Here's the drawing with two shaded views (mm, measured from the low corner). I have some questions. A direction names the side the tool comes from. Round coordinates to 2 decimals unless told otherwise and drop trailing zeros. Loops run counter-clockwise (first coordinate to the right, second up) from the corner with the lowest first, then second, coordinate; pieces in that order, holes last. Notation, with made-up numbers: M 86,67 L 112,67 A24 ccw 112,92 Z; hole C -3,15.5 d1. An arc over 180 degrees is marked long. Answer as a JSON object with one key per item and string values.
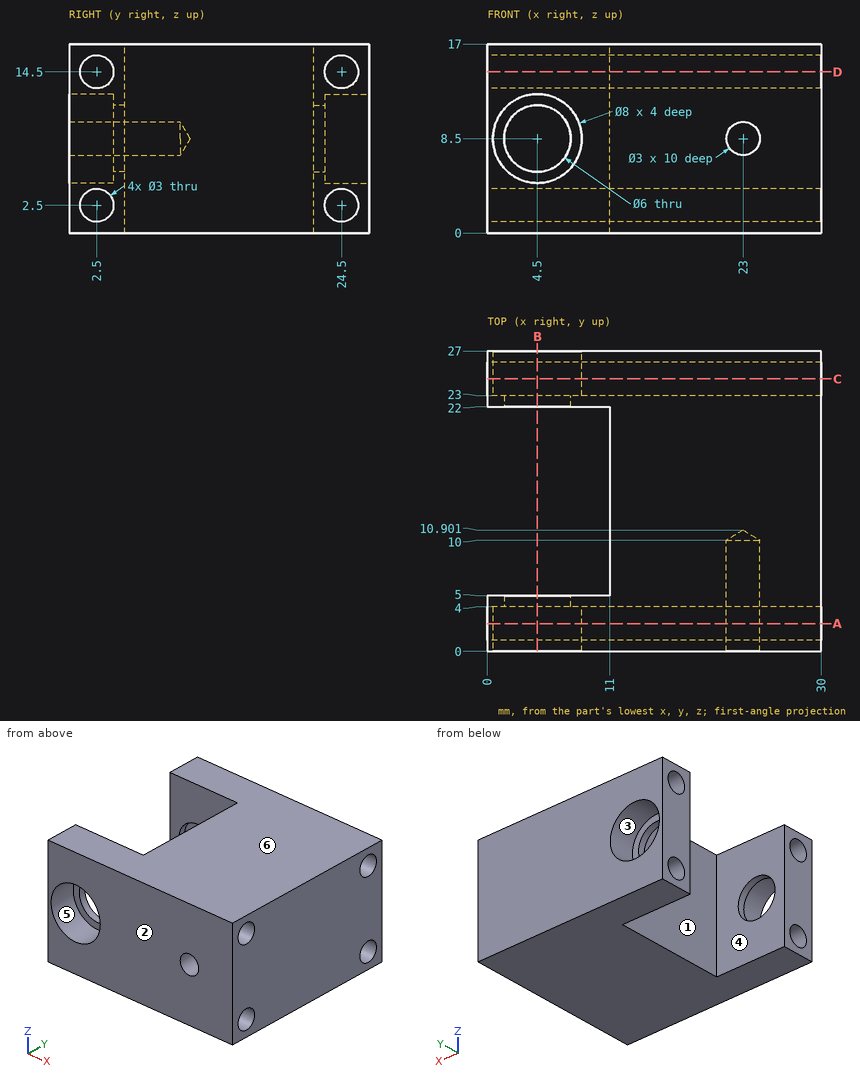
Item 1: We'd pull the mould along X, two halves only. Please class the marked faces 1, 2 and 3: +X half, -X half, draft (parallel to the pull), parting line (faces both ways), or undercut.
Solution:
{"face 1": "-X half", "face 2": "draft", "face 3": "undercut"}
Item 2: I want a section at B-B on x = 4.5. List the corners of the cut face in (y, z) for me.
Solution:
{"outline": "M 0,0 L 5,0 L 5,5.5 L 4,5.5 L 4,4.5 L 0,4.5 Z; M 0,12.5 L 4,12.5 L 4,11.5 L 5,11.5 L 5,17 L 0,17 Z; M 22,0 L 27,0 L 27,4.5 L 23,4.5 L 23,5.5 L 22,5.5 Z; M 22,11.5 L 23,11.5 L 23,12.5 L 27,12.5 L 27,17 L 22,17 Z; hole C 2.5,2.5 d3; hole C 2.5,14.5 d3; hole C 24.5,2.5 d3; hole C 24.5,14.5 d3"}
Item 3: For P1, Ø1.8, axis at x = 23, z = 8.5, coming from the -Y side; P2, Ø7, axis at x = 4.5, z = 8.5, coming from the -Y side, each with a flat end and sliding along its axis, tell me the tip position at first contact or that it passes through.
Solution:
{"P1": "stops at y = 10.36", "P2": "stops at y = 4"}
Item 4: I want a section at D-D on z = 14.5. List the corners of the cut face in (x, y) for me.
Solution:
{"outline": "M 0,0 L 30,0 L 30,1 L 0,1 Z; M 0,4 L 30,4 L 30,23 L 0,23 L 0,22 L 11,22 L 11,5 L 0,5 Z; M 0,26 L 30,26 L 30,27 L 0,27 Z"}
Item 5: I want a section at A-A on y = 2.5. List the corners of the cut face in (x, z) for me.
Solution:
{"outline": "M 0,0 L 30,0 L 30,1 L 0,1 Z; M 0,4 L 30,4 L 30,13 L 0,13 Z; M 0,16 L 30,16 L 30,17 L 0,17 Z; hole C 4.5,8.5 d8; hole C 23,8.5 d3"}
Item 6: I want a section at C-C on y = 24.5. List the corners of the cut face in (x, z) for me.
Solution:
{"outline": "M 0,0 L 30,0 L 30,1 L 0,1 Z; M 0,4 L 30,4 L 30,13 L 0,13 Z; M 0,16 L 30,16 L 30,17 L 0,17 Z; hole C 4.5,8.5 d8"}
Item 7: For the marked faces 4, 5 and 6, which set-ups out of +Z, -Z, +X, -X, +Y, -Y let a thin tool reach every point of the face, with its end or its side?
Solution:
{"face 4": "+Z, -Z, -X", "face 5": "-Y", "face 6": "+Z, +X, -X, +Y, -Y"}
Item 8: If I drill on L1, parallel to Z at x = 11, y = 2.5; L2, parallel to Y at x = 7.75, z = 11; L3, parallel to Z at x = 4.5, y = 2.4, over which ranges is the centre line in solid material (lowest first)? Write a range as from..to.
Solution:
{"L1": "z = 0..1, 4..13, 16..17", "L2": "y = 0..5, 22..27", "L3": "z = 0..1, 4..4.5, 12.5..13, 16..17"}
